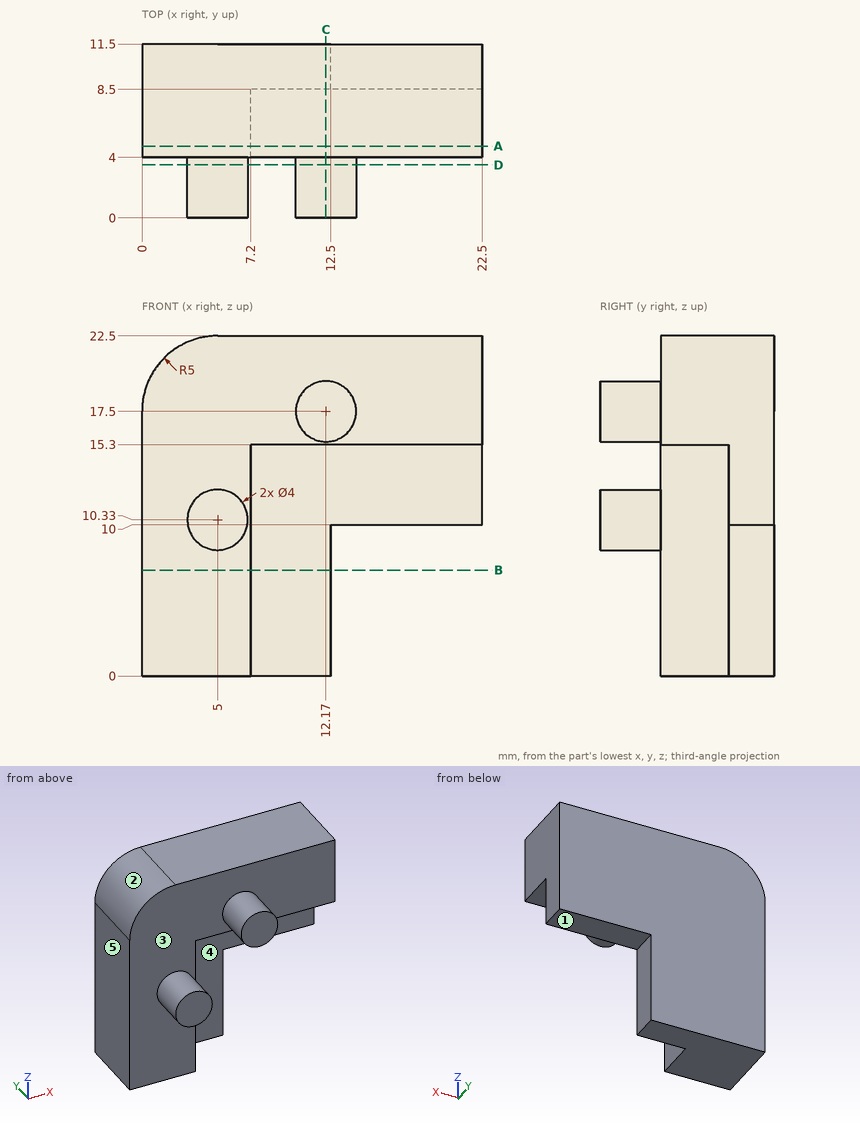
For this review, use the dimensioned drawing (mm, ordinates from the lowest corner) and the shaded views. A direction names the side the tool comes from. Give positions to 0.01 mm unless a question says otherwise; leave off trailing zeros. Order: outer loops, then holes, each group sorted by start corner. A loop starts at its lowest first (then second) coordinate and runs counter-clockwise, first axis right, second up. Notation, with made-up numbers: M 61,23 L 65,23 A18 cw 65,52 Z; hole C 14.25,68 d10. An arc over 180 degrees is marked long. Use one line per item in the form item = value. Start each with the question number.
Item 1: We need section D-D on y = 3.5. Give the boundary of the cut face in (x, z).
Item 2: We need section A-A on y = 4.75. Give the boundary of the cut face in (x, z).
Item 3: Insertion check: pin 1 Ø4 at (x, y) = (16, 4.5) entering from -Z; pin 2 Ø6 at (y, z) = (5, 10.5) entering from +X; pin 3 Ø7.5 at (x, z) = (16, 4) entering from -Y. Each pin has a flat end and moves straight along its axis. Give the tip position at first contact, or say it passes through.
Item 4: To check wall thickness, follow line 1 along Z through (x, y) = (4.75, 9.75); line 2 along Y through (x, z) = (14.25, 21.5); line 3 along Y through (x, z) = (8.5, 1.25). State the ranges of each line that lie inside material, in increasing order. Write a range as from..to.
Item 5: For the marked faces 1, 2, 3, 4 and 5, list the 3-axis set-ups (+Z, -Z, +X, -X, +Y, -Y) from which the entire face can be reached by the end or side of a thin tool; tool diameter is ignored.
Item 6: We need section B-B on z = 7. Give the boundary of the cut face in (x, y).
Item 7: We need section C-C on x = 12.17. Give the boundary of the cut face in (y, z), plus the area to 3 significant figures.
Completed:
q1.outline = C 5,10.33 d4; C 12.17,17.5 d4
q2.outline = M 0,0 L 7.2,0 L 7.2,15.3 L 22.5,15.3 L 22.5,22.5 L 5,22.5 A5 ccw 0,17.5 Z
q3.pin_1 = 15.3
q3.pin_2 = 7.2
q3.pin_3 = 8.5
q4.line_1 = 0..22.49
q4.line_2 = 4..11.5
q4.line_3 = 8.5..11.5
q5.face_1 = -Z, +X, +Y, -Y
q5.face_2 = +Z, -X, +Y, -Y
q5.face_3 = -Y
q5.face_4 = -Z, +X, -Y
q5.face_5 = +Z, -Z, -X, +Y, -Y
q6.outline = M 0,4 L 7.2,4 L 7.2,8.5 L 12.5,8.5 L 12.5,11.5 L 0,11.5 Z
q7.outline = M 0,15.5 L 4,15.5 L 4,15.3 L 8.5,15.3 L 8.5,0 L 11.5,0 L 11.5,22.5 L 4,22.5 L 4,19.5 L 0,19.5 Z
q7.area = 116 mm²
